```python
from build123d import *

# Parameters (mm, degrees)
F0_R     = 1.7272
F1_DEPTH = 4.7625
F3_DEPTH = 7.9375
F4_R     = 1.7272
F5_DEPTH = 7.9375


with BuildPart() as f1:
    # F0 (on Top) → F1 (new body)
    with BuildSketch(Plane.XY):
        with BuildLine():
            Line((-4.4502401135, 4.4502401135), (0, 0))
            Line((0, 0), (-79.7381539824, 0))
            Line((-79.7381539824, 0), (-77.6839886087, 1.3305217617))
            ThreePointArc((-77.6839886087, 1.3305217617), (-76.5105259182, 6.8191407537), (-81.9991449101, 7.9926034442))
            Line((-81.9991449101, 7.9926034442), (-95.3233082751, -0.6377091588))
            ThreePointArc((-95.3233082751, -0.6377091588), (-96.9717152071, -5.0936740472), (-93.1657301243, -7.9375))
            Line((-93.1657301243, -7.9375), (9.5814100757, -7.9375))
            ThreePointArc((9.5814100757, -7.9375), (13.2480569703, -5.4875248722), (12.3877401135, -1.1624199622))
            Line((12.3877401135, -1.1624199622), (1.1624199622, 10.0629001892))
            ThreePointArc((1.1624199622, 10.0629001892), (-4.4502401135, 10.0629001892), (-4.4502401135, 4.4502401135))
        make_face()
        with Locations((-93.1657301243, -3.96875)):
            Circle(F0_R, mode=Mode.SUBTRACT)
        with Locations((9.5814100757, -3.96875)):
            Circle(F0_R, mode=Mode.SUBTRACT)
        with Locations((-79.8415667594, 4.661562603)):
            Circle(F0_R, mode=Mode.SUBTRACT)
        with Locations((-1.6439100757, 7.2565701513)):
            Circle(F0_R, mode=Mode.SUBTRACT)
    extrude(amount=F1_DEPTH)

    # F2 (on face) → F3 (join, through all)
    with BuildSketch(Plane.XZ.offset(7.9375)):
        with BuildLine():
            Line((-78.8949317151, 4.7625), (-72.1597396243, 4.7625))
            Line((-72.1597396243, 4.7625), (-65.4245475335, 4.7625))
            Line((-65.4245475335, 4.7625), (-68.7921435789, 8.1300960454))
            ThreePointArc((-68.7921435789, 8.1300960454), (-72.1597396243, 9.525), (-75.5273356697, 8.1300960454))
            Line((-75.5273356697, 8.1300960454), (-78.8949317151, 4.7625))
        make_face()
        with BuildLine():
            Line((-18.1597725151, 4.7625), (-11.4245804243, 4.7625))
            Line((-11.4245804243, 4.7625), (-4.6893883335, 4.7625))
            Line((-4.6893883335, 4.7625), (-8.0569843789, 8.1300960454))
            ThreePointArc((-8.0569843789, 8.1300960454), (-11.4245804243, 9.525), (-14.7921764697, 8.1300960454))
            Line((-14.7921764697, 8.1300960454), (-18.1597725151, 4.7625))
        make_face()
    extrude(amount=-F3_DEPTH)

    # F4 (on face) → F5 (cut, through all)
    with BuildSketch(Plane.XZ.offset(7.9375)):
        with Locations((-72.1597396243, 4.7625)):
            Circle(F4_R)
        with Locations((-11.4245804243, 4.7625)):
            Circle(F4_R)
    extrude(amount=-F5_DEPTH, mode=Mode.SUBTRACT)


solid = f1.part
```
Read the model definition and answer for the solid it produces. Units are mm, in the model's axes. A direction names the side the tool comes from. Round coordinates to 2 decimals unless told otherwise and drop trailing zeros. Write each loop counter-clockwise with the first axis right and the second up, starting at its lowest first coordinate (ties: lowest second). Pieces come first, ordered by that corner, then holes. Notation, with made-up numbers: (0, 55) - (20, 55) arc R21 ccw to (20, 92) - close; hole circle Ø7 at (68, 62.5). An arc over 180 degrees is marked (long way). One line per item, written item: value.
Q1. Each of these flat-tipped pins is pushed along its axis until it touches: P1, Ø3, axis at y = 9, z = 2.5, coming from the +X side; P2, Ø1, axis at y = 1.5, z = 4.5, coming from the -X side; P3, Ø1.5, axis at x = -44, y = -5.5, coming from the +Z side. Where does it stop, or does it pass through?
The answers:
P1: stops at x = 3.73
P2: stops at x = -92.79
P3: stops at z = 4.76
Q2. For a pull along Z with two mould halves and no side action, classify faces 1 (the cylindrical face through (-11.649, -4.024, 6.475)), 2 (the cylindrical face through (-78.2, 5.2, 2.3)), 3 (the flat face through (2, 0, 4.762)) as pulls with the +Z half, pulls with the -Z half, needs draft (parallel to the pull), parting line crosses it, or undercut.
The answers:
face 1: undercut
face 2: needs draft
face 3: pulls with the +Z half
Q3. Find section B-B (x = -30). Determine the outline of the cut face in (y, z).
The answers:
outline: (-7.94, 0) - (0, 0) - (0, 4.76) - (-7.94, 4.76) - close
Q4. Straight lines are drawn through the part: line 1 (X direction, y = -2.5, z = 0.5); line 2 (X direction, y = 7.5, z = 4.5); line 3 (X direction, y = -5.25, z = 6). For each, find the intervals that lie inside material, in ascending order. Write a range as from..to.
The answers:
line 1: x = -96.85..-94.07, -92.26..8.67, 10.49..13.27
line 2: x = -82.76..-77.07, -5.61..-3.35, 0.07..3.73
line 3: x = -77.66..-73.36, -70.95..-66.66, -16.92..-12.63, -10.22..-5.93
Q5. Find section A-A (z = 1.25). Determine the outline of the cut face in (x, y), and give its area (3 significant figures).
The answers:
outline: (-95.32, -0.64) arc R3.97 ccw to (-93.17, -7.94) - (9.58, -7.94) arc R3.97 ccw to (12.39, -1.16) - (1.16, 10.06) arc R3.97 ccw to (-4.45, 4.45) - (0, 0) - (-79.74, 0) - (-77.68, 1.33) arc R3.97 ccw to (-82, 7.99) - close; hole circle Ø3.45 at (-93.17, -3.97); hole circle Ø3.45 at (-79.84, 4.66); hole circle Ø3.45 at (-1.64, 7.26); hole circle Ø3.45 at (9.58, -3.97)
area: 1,030 mm2
Q6. Which of the six approach directions +Z, -Z, +X, -X, +Y, -Y give full straight-line access (tool end or side, diameter ignored) to faces 4 (the flat face through (-67.08, -4.02, 6.42)), 5 (the cylindrical face through (-2.02, 5.57, 2.35))?
The answers:
face 4: +Z, +Y, -Y
face 5: +Z, -Z
